from build123d import *

# Parameters (mm, degrees)
SKETCH1_W                      = 57.15
SKETCH1_H                      = 51.562
SKETCH1_R                      = 21.59
BOSS_EXTRUDE1_DEPTH            = 2.286
F_3_16_0_1875_DIAMETER_HOLE1_D = 4.7625
CHAMFER1_SIZE                  = 2.286


with BuildPart() as part:
    # Sketch1 → Boss-Extrude1 (new body)
    with BuildSketch(Plane.XY):
        Rectangle(SKETCH1_W, SKETCH1_H)
        Circle(SKETCH1_R, mode=Mode.SUBTRACT)
    extrude(amount=BOSS_EXTRUDE1_DEPTH)

    # 3/16 (0.1875) Diameter Hole1 (through all)
    with Locations(Plane.XY.offset(2.286)):
        with Locations((21.336, 21.336), (-21.336, 21.336), (-21.336, -21.336), (21.336, -21.336)):
            Hole(F_3_16_0_1875_DIAMETER_HOLE1_D / 2)

    # Chamfer1
    chamfer1_edges = [part.edges().sort_by_distance(p)[0] for p in [
        (-28.575, 25.781, 1.143),
        (28.575, 25.781, 1.143),
        (28.575, -25.781, 1.143),
        (-28.575, -25.781, 1.143),
    ]]
    chamfer(chamfer1_edges, length=CHAMFER1_SIZE)


solid = part.part
The listing builds one solid part. Answer for the finished solid, in the listing's coordinates (mm). Coordinates: 2 decimals unless noted, no trailing zeros. Order: outer loops, then holes, each group sorted by start corner. A loop starts at its lowest first (then second) coordinate and runs counter-clockwise, first axis right, second up. Notation, with made-up numbers: (62.5, 24.5) -> (118.5, 24.5) arc R4 cw to (118.5, 31.5) -> close; hole circle Ø8 at (68, 0). An arc over 180 degrees is marked (long way). Answer in a Markdown table with one row per item. Add a question column.
Item 1: Find section B-B (x = 0). Write down the section's boundary in (y, z), then the cut area to 3 significant figures.
Item 2: Find the intervals of material crossed by L1, parallel to X at y = 23, z = 1.05 (3 decimals); L2, parallel to X at y = -19.5, z = 1.3 (3 decimals); L3, parallel to Y at x = 0, z = 1.3, in increasing order. Write a range as from..to.
Item 3: Find section C-C (z = 1.1). Write down the section's boundary in (x, y) (1 decimal), then the cut area to 3 significant figures.
Item 4: This flat-tipped pin is pushed along its axis until it touches: P1, Ø2, axis at x = -21.5, y = 9, coming from the -Z side. Where does it stop, or does it pass through?
Item 5: Determine the mould class of faces 1 (the face through (27.45, -24.62, 1.13)), 2 (the face through (19.065, 22.051, 1.127)), 3 (the face through (-13, 18, 0)), 4 (the face through (-15.913, 14.592, 1.127)) for opening direction Y: +Y half, -Y half, draft (parallel to the pull), parting line (faces both ways), or undercut.
Item 6: Find section A-A (y = 0). Write down the section's boundary in (x, z) (3 decimals).
Result set:
| question | item | result |
|---|---|---|
| 1 | outline | (-25.78, 0) -> (-21.59, 0) -> (-21.59, 2.29) -> (-25.78, 2.29) -> close; (21.59, 0) -> (25.78, 0) -> (25.78, 2.29) -> (21.59, 2.29) -> close |
| 1 | area | 19.2 mm² |
| 2 | L1 | x = -28.575..-23.039, -19.633..19.633, 23.039..28.575 |
| 2 | L2 | x = -28.575..-22.852, -19.82..-9.267, 9.267..19.82, 22.852..28.575 |
| 2 | L3 | y = -25.78..-21.59, 21.59..25.78 |
| 3 | outline | (-28.6, -23.5) -> (-26.3, -25.8) -> (26.3, -25.8) -> (28.6, -23.5) -> (28.6, 23.5) -> (26.3, 25.8) -> (-26.3, 25.8) -> (-28.6, 23.5) -> close; hole circle Ø4.8 at (-21.3, -21.3); hole circle Ø4.8 at (-21.3, 21.3); hole circle Ø43.2 at (0, 0); hole circle Ø4.8 at (21.3, -21.3); hole circle Ø4.8 at (21.3, 21.3) |
| 3 | area | 1,400 mm² |
| 4 | P1 | stops at z = 0 |
| 5 | face 1 | -Y half |
| 5 | face 2 | undercut |
| 5 | face 3 | draft |
| 5 | face 4 | undercut |
| 6 | outline | (-28.575, 0) -> (-21.59, 0) -> (-21.59, 2.286) -> (-28.575, 2.286) -> close; (21.59, 0) -> (28.575, 0) -> (28.575, 2.286) -> (21.59, 2.286) -> close |
